from build123d import *

# Parameters (mm, degrees)
F2_DEPTH = 400
F3_DEPTH = 550
F0_W     = 100
F0_H     = 900
F4_DEPTH = 700


# Not quite as in the source:
# - the program builds the solid bodies; features that only make, move or delete a surface that nothing else refers to are left out


with BuildPart() as f2:
    # F0 (on Top) → F2 (new body)
    with BuildSketch(Plane.XY):
        Polygon((2869.0189361572, -358.3241462708), (969.0189361572, -358.3241462708), (969.0189361572, -1258.3241462708), (2569.0189361572, -1258.3241462708), align=None)
    extrude(amount=F2_DEPTH)

    # F0 (on Top) → F3 (join)
    with BuildSketch(Plane.XY):
        Polygon((2869.0189361572, -1258.3241462708), (2869.0189361572, -358.3241462708), (2569.0189361572, -1258.3241462708), align=None)
    extrude(amount=F3_DEPTH)

    # F0 (on Top) → F4 (join)
    with BuildSketch(Plane.XY):
        with Locations((2919.0189361572, -808.3241462708)):
            Rectangle(F0_W, F0_H)
    extrude(amount=F4_DEPTH)


solid = f2.part
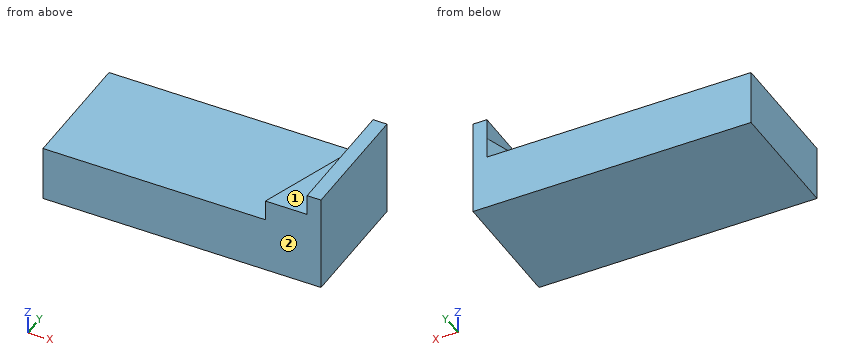
CAD build for the part. Positions are in the model's coordinates, mm. Face numbers are marked on the shaded views. A direction names the side the tool comes from. Round coordinates to 2 decimals unless told otherwise and drop trailing zeros. Write each loop counter-clockwise with the first axis right and the second up, starting at its lowest first coordinate (ties: lowest second). Pieces come first, ordered by that corner, then holes. Notation, with made-up numbers: (69.5, 13) -> (115.5, 13) arc R33 ccw to (115.5, 44) -> close; hole circle Ø3 at (34.5, -2). An arc over 180 degrees is marked (long way). Answer as a JSON object with one key per item and string values.
(1) Pin check, flat tips, straight feed: P1, Ø4, axis at x = 1301.5, y = -987.5, coming from the +Z side; P2, Ø10, axis at x = 1376, z = 403.5, coming from the +Y side. Stop position of each tip, or through.
Reported:
{"P1": "stops at z = 400", "P2": "stops at y = -358.32"}
(2) Probe probe 1 along Z at (x, y) = (1318.5, -754); probe 2 along X at (y, z) = (-489.5, 612); probe 3 along X at (y, z) = (-528, 516). List the from-to ranges inside material, lowest first. Write a range as [from, to].
Reported:
{"probe 1": "z = [0, 400]", "probe 2": "x = [2869.02, 2969.02]", "probe 3": "x = [2812.46, 2969.02]"}
(3) Band-saw the part on C-C, the plane z = 583. List the corners of the cut face in (x, y), then the cut area to 3 significant figures.
Reported:
{"outline": "(2869.02, -1258.32) -> (2969.02, -1258.32) -> (2969.02, -358.32) -> (2869.02, -358.32) -> close", "area": "90,000 mm^2"}
(4) Band-saw the part on B-B, the plane x = 1767.5. List the corners of the cut face in (y, z), then the cut area to 3 significant figures.
Reported:
{"outline": "(-1258.32, 0) -> (-358.32, 0) -> (-358.32, 400) -> (-1258.32, 400) -> close", "area": "360,000 mm^2"}
(5) Band-saw the part on A-A, the plane y = -655.5. List the corners of the cut face in (x, z).
Reported:
{"outline": "(969.02, 0) -> (2969.02, 0) -> (2969.02, 700) -> (2869.02, 700) -> (2869.02, 550) -> (2769.96, 550) -> (2769.96, 400) -> (969.02, 400) -> close"}
(6) Which spindle directions (+Z, -Z, +X, -X, +Y, -Y) get a long thin tool onto all of the face, cutting with end or side? Do the marked faces 1 and 2. Say none if no direction does.
Reported:
{"face 1": "+Z, -X, +Y, -Y", "face 2": "+Z, -Z, +X, -X, -Y"}
(7) Band-saw the part on D-D, the plane y = -746. List the corners of the cut face in (x, z), then the cut area to 3 significant figures.
Reported:
{"outline": "(969.02, 0) -> (2969.02, 0) -> (2969.02, 700) -> (2869.02, 700) -> (2869.02, 550) -> (2739.79, 550) -> (2739.79, 400) -> (969.02, 400) -> close", "area": "849,000 mm^2"}
